Design review of the part built by this model. Coordinates are the model's own, in mm. A direction names the side the tool comes from. Coordinates: 2 decimals unless noted, no trailing zeros. Write each loop counter-clockwise with the first axis right and the second up, starting at its lowest first coordinate (ties: lowest second). Pieces come first, ordered by that corner, then holes. Notation, with made-up numbers: (2.5, 85) - (60.5, 85) arc R36 cw to (60.5, 120) - close; hole circle Ø11 at (-27.5, 43). An arc over 180 degrees is marked (long way). Answer as a JSON object with one key per item and string values.
```python
from build123d import *

# Parameters (mm, degrees)
SKETCH1_W            = 60
SKETCH1_H            = 110
BOSS_EXTRUDE1_DEPTH  = 2
SKETCH2_W            = 60
SKETCH2_H            = 110
SKETCH2_W_2          = 56
SKETCH2_H_2          = 106
BOSS_EXTRUDE2_DEPTH  = 50
SKETCH3_W            = 60
SKETCH3_H            = 30
BOSS_EXTRUDE3_DEPTH  = 2
BOSS_EXTRUDE4_DEPTH  = 50
SKETCH5_R            = 2.486759959
CUT_EXTRUDE1_DEPTH   = 30
CUT_SWEEP1_PROFILE_R = 0.5
SKETCH43_W           = 7.5
SKETCH43_H           = 140
BOSS_EXTRUDE7_DEPTH  = 3
SKETCH55_W           = 7.1
SKETCH55_H           = 8
BOSS_EXTRUDE10_DEPTH = 20.2
SKETCH56_R           = 2
CUT_EXTRUDE3_DEPTH   = 46.2
SKETCH59_R           = 2
CUT_EXTRUDE4_DEPTH   = 49.2
SKETCH60_R           = 2.925
BOSS_EXTRUDE11_DEPTH = 4
SKETCH61_R           = 2.925
BOSS_EXTRUDE12_DEPTH = 4
SKETCH62_R           = 1.025
CUT_EXTRUDE5_DEPTH   = 10
BOSS_EXTRUDE13_DEPTH = 25
SKETCH64_R           = 2.925
BOSS_EXTRUDE14_DEPTH = 4
BOSS_EXTRUDE15_DEPTH = 25
SKETCH66_R           = 2.925
BOSS_EXTRUDE16_DEPTH = 4


with BuildPart() as part:
    # Sketch1 → Boss-Extrude1 (new body)
    with BuildSketch(Plane(origin=(0, 0, 0), x_dir=(1, 0, 0), z_dir=(0, 1, 0))):
        Rectangle(SKETCH1_W, SKETCH1_H)
    extrude(amount=BOSS_EXTRUDE1_DEPTH)

    # Sketch2 → Boss-Extrude2 (add)
    with BuildSketch(Plane(origin=(0, 2, 0), x_dir=(1, 0, 0), z_dir=(0, 1, 0))):
        Rectangle(SKETCH2_W, SKETCH2_H)
        Rectangle(SKETCH2_W_2, SKETCH2_H_2, mode=Mode.SUBTRACT)
    extrude(amount=BOSS_EXTRUDE2_DEPTH)

    # Sketch3 → Boss-Extrude3 (add)
    with BuildSketch(Plane(origin=(0, 0, 0), x_dir=(1, 0, 0), z_dir=(0, 1, 0))):
        with Locations((0, -70)):
            Rectangle(SKETCH3_W, SKETCH3_H)
    extrude(amount=BOSS_EXTRUDE3_DEPTH)

    # Sketch4 → Boss-Extrude4 (add)
    with BuildSketch(Plane(origin=(0, 2, 0), x_dir=(1, 0, 0), z_dir=(0, 1, 0))):
        Polygon((-28, -55), (-30, -55), (-30, -85), (30, -85), (30, -55), (28, -55), (28, -83), (-28, -83), align=None)
    extrude(amount=BOSS_EXTRUDE4_DEPTH)

    # Sketch5 → Cut-Extrude1 (cut)
    with BuildSketch(Plane.XY.offset(55)):
        with Locations((0, 15.890944925)):
            Circle(SKETCH5_R)
    extrude(amount=-CUT_EXTRUDE1_DEPTH, mode=Mode.SUBTRACT)

    # Cut-Sweep1: sweep along a path in Sketch6
    with BuildLine(Plane(origin=(0, 52, 0), x_dir=(1, 0, 0), z_dir=(0, 1, 0))) as cut_sweep1_path:
        Line((-29, 54), (-29, -84))
        Line((-29, -84), (29, -84))
        Line((29, -84), (29, 54))
        Line((29, 54), (-29, 54))
    # Cut-Sweep1 profile (on start of the path) → Cut-Sweep1 (sweep, cut)
    with BuildSketch(Plane(origin=(-29, 52, -54), x_dir=(1, 0, 0), z_dir=(0, 0, 1))):
        Circle(CUT_SWEEP1_PROFILE_R)
    sweep(path=cut_sweep1_path.line, transition=Transition.RIGHT, mode=Mode.SUBTRACT)

    # Sketch43 → Boss-Extrude7 (add)
    with BuildSketch(Plane.XZ):
        with Locations((33.75, 15)):
            Rectangle(SKETCH43_W, SKETCH43_H)
        Polygon((-30, -55), (-37.5, -55), (-37.5, 85), (-30, 85), (-30, 55), align=None)
    extrude(amount=-BOSS_EXTRUDE7_DEPTH)

    # Sketch55 → Boss-Extrude10 (add)
    with BuildSketch(Plane.XZ):
        with Locations((-33.95, 65.9)):
            Rectangle(SKETCH55_W, SKETCH55_H)
        Polygon((9.6, 69.9), (9.6, 61.9), (25.881976889, 61.9), (25.881976889, 77), (37.5, 77), (37.5, 85), (16.7, 85), (16.7, 69.9), align=None)
        with Locations((33.95, -35.9)):
            Rectangle(SKETCH55_W, SKETCH55_H)
        Polygon((-9.6, -39.9), (-9.6, -31.9), (-24.7, -31.9), (-24.7, -47), (-37.5, -47), (-37.5, -55), (-16.7, -55), (-16.7, -39.9), align=None)
    extrude(amount=BOSS_EXTRUDE10_DEPTH)

    # Sketch56 → Cut-Extrude3 (cut)
    with BuildSketch(Plane.XY.offset(85)):
        with Locations((-34.9, -15.1)):
            Circle(SKETCH56_R)
        with Locations((-34.9, -5.1)):
            Circle(SKETCH56_R)
        with Locations((14.1, -15.1)):
            Circle(SKETCH56_R)
        with Locations((14.1, -5.1)):
            Circle(SKETCH56_R)
    extrude(amount=-CUT_EXTRUDE3_DEPTH, mode=Mode.SUBTRACT)

    # Sketch59 → Cut-Extrude4 (cut)
    with BuildSketch(Plane(origin=(0, 0, -55), x_dir=(-1, 0, 0), z_dir=(0, 0, -1))):
        with Locations((-34.9, -15.1)):
            Circle(SKETCH59_R)
        with Locations((-34.9, -5.1)):
            Circle(SKETCH59_R)
        with Locations((14.1, -5.1)):
            Circle(SKETCH59_R)
        with Locations((14.1, -15.1)):
            Circle(SKETCH59_R)
    extrude(amount=-CUT_EXTRUDE4_DEPTH, mode=Mode.SUBTRACT)

    # Sketch60 → Boss-Extrude11 (add)
    with BuildSketch(Plane(origin=(0, 0, -55), x_dir=(-1, 0, 0), z_dir=(0, 0, -1))):
        with Locations((20.55, -10.1)):
            Circle(SKETCH60_R)
    extrude(amount=BOSS_EXTRUDE11_DEPTH)

    # Sketch61 → Boss-Extrude12 (add)
    with BuildSketch(Plane.XY.offset(85)):
        with Locations((20.55, -10.1)):
            Circle(SKETCH61_R)
    extrude(amount=BOSS_EXTRUDE12_DEPTH)

    # Sketch62 → Cut-Extrude5 (cut)
    with BuildSketch(Plane.XY.offset(85)):
        with Locations((0, 27.5)):
            Circle(SKETCH62_R)
    extrude(amount=-CUT_EXTRUDE5_DEPTH, mode=Mode.SUBTRACT)

    # Sketch63 → Boss-Extrude13 (add)
    with BuildSketch(Plane.XZ.offset(20.2)):
        Polygon((16.7, 69.9), (9.6, 69.9), (9.6, 61.9), (25.881976889, 61.9), (25.881976889, 77), (37.5, 77), (37.5, 85), (16.7, 85), align=None)
    extrude(amount=BOSS_EXTRUDE13_DEPTH)

    # Sketch64 → Boss-Extrude14 (add)
    with BuildSketch(Plane.XY.offset(85)):
        with Locations((20.55, -40.1)):
            Circle(SKETCH64_R)
    extrude(amount=BOSS_EXTRUDE14_DEPTH)

    # Sketch65 → Boss-Extrude15 (add)
    with BuildSketch(Plane.XZ.offset(20.2)):
        Polygon((-16.7, -39.9), (-9.6, -39.9), (-9.6, -31.9), (-24.7, -31.9), (-24.7, -47), (-37.5, -47), (-37.5, -55), (-16.7, -55), align=None)
    extrude(amount=BOSS_EXTRUDE15_DEPTH)

    # Sketch66 → Boss-Extrude16 (add)
    with BuildSketch(Plane(origin=(0, 0, -55), x_dir=(-1, 0, 0), z_dir=(0, 0, -1))):
        with Locations((20.55, -40.1)):
            Circle(SKETCH66_R)
    extrude(amount=BOSS_EXTRUDE16_DEPTH)


solid = part.part
```
(1) Take a section at D-D, the plane z = -21. Write out the cut boundary in (x, y).
Solved:
{"outline": "(-37.5, 0) - (37.5, 0) - (37.5, 3) - (30, 3) - (30, 52) - (29.5, 52) arc R0.5 cw to (28.5, 52) - (28, 52) - (28, 2) - (-28, 2) - (-28, 52) - (-28.5, 52) arc R0.5 cw to (-29.5, 52) - (-30, 52) - (-30, 3) - (-37.5, 3) - close"}
(2) Take a section at B-B, the plane x = -34.9. Write out the cut boundary in (y, z), and give its area (3 significant figures).
Solved:
{"outline": "(-45.2, -55) - (3, -55) - (3, 85) - (0, 85) - (0, 69.9) - (-3.1, 69.9) - (-3.1, 61.9) - (0, 61.9) - (0, -47) - (-45.2, -47) - close; (-20.2, 61.9) - (-17.1, 61.9) - (-17.1, 69.9) - (-20.2, 69.9) - close; (-13.1, 61.9) - (-7.1, 61.9) - (-7.1, 69.9) - (-13.1, 69.9) - close", "area": "879 mm^2"}
(3) Take a section at A-A, the plane y = 9. Write out the cut boundary in (x, z), and give its area (3 significant figures).
Solved:
{"outline": "(-30, -55) - (30, -55) - (30, 85) - (-30, 85) - close; hole (-28, -53) - (28, -53) - (28, 53) - (-28, 53) - close; hole (-28, 55) - (28, 55) - (28, 83) - (-28, 83) - close", "area": "896 mm^2"}
(4) To check wall thickness, follow line 1 (Z direction, x = -24.5, y = 26.5); line 2 (Y direction, x = -14.1, z = -34.5); line 3 (X direction, y = 41.5, z = 14). State the ranges of each line that lie inside material, in increasing order. Write a range as from..to.
Solved:
{"line 1": "z = -55..-53, 53..55, 83..85", "line 2": "y = -45.2..-17.1, -13.1..-7.1, -3.1..2", "line 3": "x = -30..-28, 28..30"}
(5) For pin 1 (15 mm diameter, centred on x = -5, y = 32.5, fed in from +Z); pin 2 (5 mm diameter, centred on x = -14.1, y = -5.1, fed in from -Z); pin 3 (1.5 mm diameter, centred on x = -4, z = 51, fed in from +Y), all flat-tipped, find the tip position at first contact; note any pin that passes through.
Solved:
{"pin 1": "stops at z = 85", "pin 2": "stops at z = -39.9", "pin 3": "stops at y = 2"}
(6) Tool access review of faces 5 (the face through (34, -10, -39.9)), 6 (the face through (-9.6, -22, -36)), 7 (the face through (-34, -20.2, 66)): name each direction out of +Z, -Z, +X, -X, +Y, -Y from which nothing blocks a thin tool from reaching the whole face with its end or side.
Solved:
{"face 5": "-Z, +X, -Y", "face 6": "+Z, -Z, -Y", "face 7": "+Z, -X, -Y"}
(7) Take a section at C-C, the plane y = -31. Write out the cut boundary in (x, z).
Solved:
{"outline": "(-37.5, -55) - (-16.7, -55) - (-16.7, -39.9) - (-9.6, -39.9) - (-9.6, -31.9) - (-24.7, -31.9) - (-24.7, -47) - (-37.5, -47) - close; (9.6, 61.9) - (25.88, 61.9) - (25.88, 77) - (37.5, 77) - (37.5, 85) - (16.7, 85) - (16.7, 69.9) - (9.6, 69.9) - close"}
(8) The part is to be moulded in two halves that separate along X. For faces 1 (the face through (21, -10, 89)), 2 (the face through (30.4, -10, -36)), 3 (the face through (23.25, -11.22, 86.97)), 4 (the face through (-12.626, -3.748, -35.956)), say which applies: pulls with the +X half, pulls with the -X half, needs draft (parallel to the pull), parting line crosses it, or undercut.
Solved:
{"face 1": "needs draft", "face 2": "undercut", "face 3": "parting line crosses it", "face 4": "undercut"}
